from build123d import *

# Parameters (mm, degrees)
PAD_DEPTH       = 11
SKETCH001_W     = 20
SKETCH001_H     = 20
POCKET_DEPTH    = 2
POCKET001_DEPTH = 8


with BuildPart() as part:
    # Sketch → Pad (new body, symmetric)
    with BuildSketch(Plane.XZ):
        Polygon((-11, 0), (11, 0), (11, 3), (4, 6), (-11, 6), align=None)
    extrude(amount=PAD_DEPTH, both=True)

    # Sketch001 → Pocket (cut)
    with BuildSketch(Plane.XY):
        Rectangle(SKETCH001_W, SKETCH001_H)
    extrude(amount=POCKET_DEPTH, mode=Mode.SUBTRACT)

    # Sketch002 → Pocket001 (cut, symmetric)
    with BuildSketch(Plane.XZ):
        Polygon((-8, -1), (-8, 5), (3.794742, 5), (8, 3.197747), (8, -1), align=None)
    extrude(amount=POCKET001_DEPTH, both=True, mode=Mode.SUBTRACT)


solid = part.part
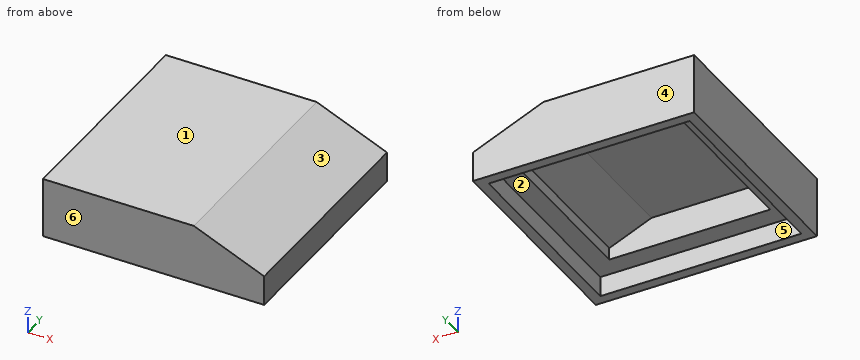
The listing builds one solid part. Answer for the finished solid, in the listing's coordinates (mm). Face numbers are marked on the shaded views. A direction names the side the tool comes from. Give positions to 0.01 mm unless a question says otherwise; leave off trailing zeros. Loops run counter-clockwise (first coordinate to the right, second up) from the corner with the lowest first, then second, coordinate; pieces in that order, holes last. Notation, with made-up numbers: (-9.5, 28.25) - (13.5, 28.25) arc R24 cw to (13.5, 43.25) - close; hole circle Ø5 at (-26, 50.5). An arc over 180 degrees is marked (long way). Use one line per item in the form item = value.
1. Section A-A on y = -2 is taken. Give the vertices of the cut face in (x, z), then the cut area to 3 significant figures.
Calculated:
outline = (-11, 0) - (-10, 0) - (-10, 2) - (-8, 2) - (-8, 5) - (3.79, 5) - (8, 3.2) - (8, 2) - (10, 2) - (10, 0) - (11, 0) - (11, 3) - (4, 6) - (-11, 6) - close
area = 37.3 mm^2
2. Find the intervals of material crossed by line 1 along Y through (x, z) = (-2, 4.9); line 2 along Y through (x, z) = (-9, 0.8), in increasing order. Write a range as [from, to].
Calculated:
line_1 = [-11, -8], [8, 11]
line_2 = [-11, -10], [10, 11]
3. Given pin 1 Ø2 at (x, y) = (2.5, -7.5) entering from -Z; pin 2 Ø3.5 at (x, y) = (-2, 2.5) entering from -Z, each flat-ended and moving along its own axis, determine where each tip first touches the part or whether it passes through.
Calculated:
pin_1 = 2
pin_2 = 5
4. Section C-C on x = -4.5 is taken. Give the vertices of the cut face in (y, z).
Calculated:
outline = (-11, 0) - (-10, 0) - (-10, 2) - (-8, 2) - (-8, 5) - (8, 5) - (8, 2) - (10, 2) - (10, 0) - (11, 0) - (11, 6) - (-11, 6) - close
5. Which of the six approach directions +Z, -Z, +X, -X, +Y, -Y give full straight-line access (tool end or side, diameter ignored) to the marked faces 1 and 2?
Calculated:
face_1 = +Z, +X, -X, +Y, -Y
face_2 = -Z
6. Section B-B on z = 1.6 is taken. Give the vertices of the cut face in (x, y), then the cut area to 3 significant figures.
Calculated:
outline = (-11, -11) - (11, -11) - (11, 11) - (-11, 11) - close; hole (-10, -10) - (10, -10) - (10, 10) - (-10, 10) - close
area = 84.0 mm^2
7. Section D-D on y = -8.5 is taken. Give the vertices of the cut face in (x, z).
Calculated:
outline = (-11, 0) - (-10, 0) - (-10, 2) - (10, 2) - (10, 0) - (11, 0) - (11, 3) - (4, 6) - (-11, 6) - close
8. The mould has two halves that part along Y. Classify the marked faces 3, 4, 5 and 6: pulls with the +Y half, pulls with the -Y half, needs draft (parallel to the pull), parting line crosses it, or undercut.
Calculated:
face_3 = needs draft
face_4 = pulls with the +Y half
face_5 = undercut
face_6 = pulls with the -Y half
